Part model, mm, in its own coordinate system. A direction names the side the tool comes from. Coordinates: 2 decimals unless noted, no trailing zeros. Order: outer loops, then holes, each group sorted by start corner. A loop starts at its lowest first (then second) coordinate and runs counter-clockwise, first axis right, second up.
```python
from build123d import *

# Parameters (mm, degrees)
F1_DEPTH = 2.54


with BuildPart() as f1:
    # F0 (on Front) → F1 (new body)
    with BuildSketch(Plane.XZ):
        with BuildLine():
            Line((20.668315, 0), (20.668315, 26.228523))
            ThreePointArc((20.668315, 26.228523), (0.17472, 47.222494), (-20.410517, 26.318373))
            ThreePointArc((-20.410517, 26.318373), (-20.409678, 26.273447), (-20.408742, 26.228523))
            Line((-20.408742, 26.228523), (-19.833371, 0))
            Line((-19.833371, 0), (-36.207609, -32.658167))
            Line((-36.207609, -32.658167), (37.04169, -32.658167))
            Line((37.04169, -32.658167), (20.668315, 0))
        make_face()
        with BuildLine():
            ThreePointArc((0.108574, 16.981143), (-9.785373, 26.78734), (0.151377, 36.550163))
            ThreePointArc((0.151377, 36.550163), (7.140778, 33.72297), (10.045348, 26.765368))
            ThreePointArc((10.045348, 26.765368), (7.125543, 19.792734), (0.108574, 16.981143))
        make_face(mode=Mode.SUBTRACT)
    extrude(amount=F1_DEPTH)

    # F2: F1 across plane


with BuildPart() as f1_1:
    add(f1.part)
    add(f1.part.mirror(Plane.YZ))


solid = f1_1.part
```
(1) Probe line 1 (X direction, y = -1.05, z = 2.5); line 2 (Z direction, x = 3, y = -0.4); line 3 (X direction, y = -2.3, z = 29). List the from-to ranges inside material, lowest first.
(2) Drop flat-ended pins along their axis: pin 1 (4 mm diameter, centred on x = 13.5, z = 8.5, fed in from +Y); pin 2 (0.8 mm diameter, centred on y = -1.5, z = 10, fed in from -X); pin 3 (1.5 mm diameter, centred on y = -1.5, z = -14.5, fed in from -X); pin 4 (1.3 mm diameter, centred on y = -2, z = 11, fed in from +X). Give the stop position or say it passes through.
(3) Slice it at B-B, the plane z = -21. Give the cut face in (x, y), then the cut area to 3 significant figures.
(4) Slice it at C-C, the plane x = -16.5. Give the cut face in (y, z).
(5) Tool access for faces 1 (the face through (20.668, -1, 13)), 2 (the face through (1, -1, -32.658)), 3 (the face through (-20.668, -1, 13)): list every direction of +Z, -Z, +X, -X, +Y, -Y with a clear straight run to the whole face (end or side of a thin tool).
(6) Slice it at A-A, the plane y = -1.1. Give the cut face in (x, z), then the cut area to 3 significant figures.
Here are the results:
1. line 1: x = -20.67 to 20.67
1. line 2: z = -32.66 to 17.45, 36.08 to 47.02
1. line 3: x = -20.54 to -9.53, 9.53 to 20.54
2. pin 1: stops at y = 0
2. pin 2: stops at x = -20.67
2. pin 3: stops at x = -28.31
2. pin 4: stops at x = 20.67
3. outline: (-31.2, -2.54) - (31.2, -2.54) - (31.2, 0) - (-31.2, 0) - close
3. area: 158 mm2
4. outline: (-2.54, -32.66) - (0, -32.66) - (0, 39.09) - (-2.54, 39.09) - close
5. face 1: +Z, +X, +Y, -Y
5. face 2: -Z, +X, -X, +Y, -Y
5. face 3: +Z, -X, +Y, -Y
6. outline: (-37.04, -32.66) - (37.04, -32.66) - (20.67, 0) - (20.67, 26.23) arc R20.54 ccw to (0, 47.22) arc R20.54 ccw to (-20.67, 26.23) - (-20.67, 0) - close; hole circle Ø19.57 at (0, 26.77)
6. area: 3,350 mm2
